Design review of the part built by this model. Coordinates are the model's own, in mm. Face numbers are marked on the shaded views. Give positions to 0.01 mm unless a question says otherwise; leave off trailing zeros. Loops run counter-clockwise (first coordinate to the right, second up) from the corner with the lowest first, then second, coordinate; pieces in that order, holes last. Notation, with made-up numbers: M -22.5,66 L 5.5,66 A19 cw 5.5,82 Z; hole C -35.75,9 d9. An arc over 180 degrees is marked long. Use CSV: the item, a comma, the result in double quotes.
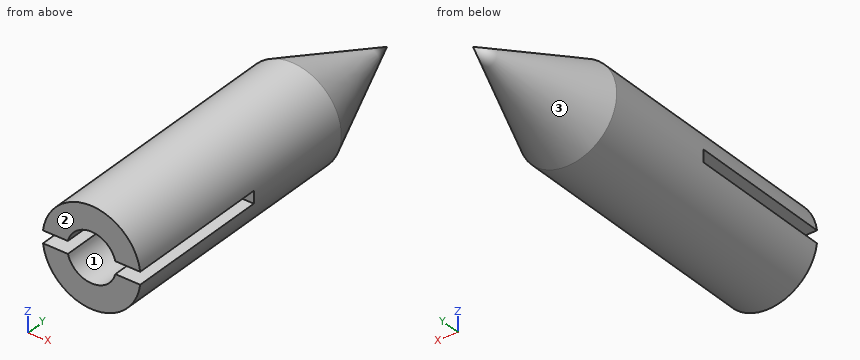
from build123d import *

# Parameters (mm, degrees)
SKETCH1_R               = 2.54
SKETCH1_R_2             = 1.27
BOSS_EXTRUDE1_DEPTH     = 11.43
BOSS_EXTRUDE2_START     = 11.43
SKETCH1_2_R             = 2.54
SKETCH1_2_R_2           = 1.27
BOSS_EXTRUDE2_DEPTH     = 2.032
CUT_EXTRUDE1_DEPTH      = 21.135007922
CUT_EXTRUDE1_DEPTH_BACK = 21.135007922
SKETCH4_W               = 0.635
SKETCH4_H               = 7.62


with BuildPart() as part:
    # Sketch1 → Boss-Extrude1 (new body)
    with BuildSketch(Plane(origin=(0, 0, 0), x_dir=(1, 0, 0), z_dir=(0, 1, 0))):
        with Locations(Location((0, 0, 0), (0, 0, 270))):
            Circle(SKETCH1_R)
        with Locations(Location((0, 0, 0), (0, 0, 270))):
            Circle(SKETCH1_R_2, mode=Mode.SUBTRACT)
    extrude(amount=BOSS_EXTRUDE1_DEPTH)

    # Sketch1<2> → Boss-Extrude2 (add)
    # profile 1 of 2: a face of its own
    with BuildSketch(Plane(origin=(0, 0, 0), x_dir=(1, 0, 0), z_dir=(0, 1, 0)).offset(BOSS_EXTRUDE2_START)):
        with Locations(Location((0, 0, 0), (0, 0, 270))):
            Circle(SKETCH1_2_R)
        with Locations(Location((0, 0, 0), (0, 0, 270))):
            Circle(SKETCH1_2_R_2, mode=Mode.SUBTRACT)
    # profile 2 of 2: a face of its own
    with BuildSketch(Plane(origin=(0, 0, 0), x_dir=(1, 0, 0), z_dir=(0, 1, 0)).offset(BOSS_EXTRUDE2_START)):
        with Locations(Location((0, 0, 0), (0, 0, 270))):
            Circle(SKETCH1_2_R_2)
    extrude(amount=BOSS_EXTRUDE2_DEPTH)

    # Sketch3 → Revolve1 (revolve)
    with BuildSketch(Plane(origin=(0, 0, 0), x_dir=(0, 0, -1), z_dir=(1, 0, 0))):
        Polygon((0, 13.462), (0, 19.812), (2.54, 13.462), align=None)
    revolve(axis=Axis((0, 13.462, 0), (0, -1, 0)))

    # Sketch4 → Cut-Extrude1 (cut, two sides: drawn at the far end of the back side and taken through both)
    with BuildSketch(Plane(origin=(0, 0, 0), x_dir=(0, 0, -1), z_dir=(1, 0, 0)).offset(-CUT_EXTRUDE1_DEPTH_BACK)):
        with Locations((0, 3.81)):
            Rectangle(SKETCH4_W, SKETCH4_H)
    extrude(amount=CUT_EXTRUDE1_DEPTH + CUT_EXTRUDE1_DEPTH_BACK, mode=Mode.SUBTRACT)


solid = part.part
(1) We need section A-A on y = 5.75. State the section outline as (x, z) points, then the cut area to 3 significant figures.
A:
outline,"M -2.52,-0.32 A2.54 ccw 2.52,-0.32 L 1.23,-0.32 A1.27 cw -1.23,-0.32 Z; M -2.52,0.32 L -1.23,0.32 A1.27 cw 1.23,0.32 L 2.52,0.32 A2.54 ccw Z"
area,"13.6 mm²"
(2) Clearance check with flat-ended pins moving along their axes: P1, Ø1.4, axis at x = -2, y = 3.5, coming from the -Z side; P2, Ø1.5, axis at x = 0.5, z = 0.5, coming from the -Y side; P3, Ø1, axis at x = 0.5, y = 14.5, coming from the +Z side; P4, Ø0.6, axis at x = 2, y = 4, coming from the +Z side. State where each tip first meets the part, or that it passes through.
A:
P1,"z = -2.18"
P2,"y = 0"
P3,"z = 2.29"
P4,"z = 1.89"
(3) The part is to be moulded in two halves that separate along Z. For the marked faces 1, 2 and 3, say which applies: released by +Z, released by -Z, zero draft, split by the parting line, or undercut.
A:
face 1,"undercut"
face 2,"zero draft"
face 3,"split by the parting line"
(4) We need section B-B on y = 12.25. State the section outline as (x, z) points, then the cut area to 3 significant figures.
A:
outline,"C 0,0 d5.08"
area,"20.3 mm²"
(5) Wall thickness on line 1 along X through (y, z) = (5, 0.45); line 2 along Z through (x, y) = (2.1, 5); line 3 along Z through (x, y) = (-1.1, 6.5): over which ranges is each line inside the solid? List them lowest first. Write a range as [from, to].
A:
line 1,"[-2.5, -1.19], [1.19, 2.5]"
line 2,"[-1.43, -0.32], [0.32, 1.43]"
line 3,"[-2.29, -0.63], [0.63, 2.29]"
(6) We need section C-C on y = 15. State the section outline as (x, z) points.
A:
outline,"C 0,0 d3.85"
